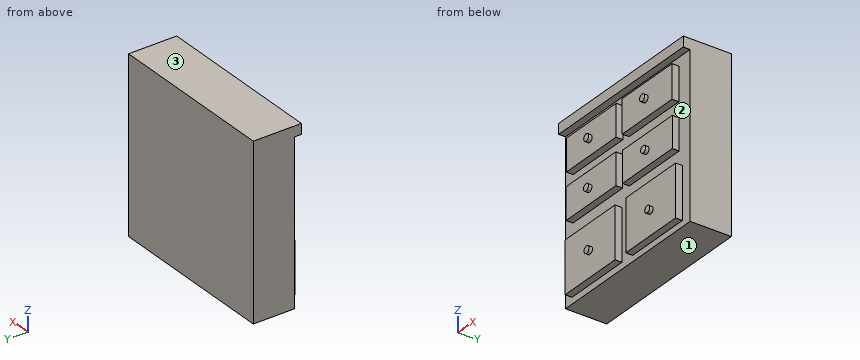
```python
from build123d import *

# Parameters (mm, degrees)
F0_W      = 50
F0_H      = 12
F1_DEPTH  = 50
F3_W      = 20
F3_H      = 9.72515
F4_DEPTH  = 2
F2_W      = 20
F2_H      = 9.250753
F5_DEPTH  = 2
F6_W      = 19.959261
F6_H      = 9.224868
F7_DEPTH  = 2
F8_W      = 20
F8_H      = 9.057143
F9_DEPTH  = 2
F10_W     = 20
F10_H     = 15
F11_DEPTH = 2
F12_W     = 20
F12_H     = 15
F13_DEPTH = 2
F14_R     = 1
F15_DEPTH = 1
F16_W     = 50
F16_H     = 3
F17_DEPTH = 2
F18_R     = 1
F19_DEPTH = 1
F20_R     = 1
F21_DEPTH = 1
F22_R     = 1
F23_DEPTH = 1
F24_R     = 1
F25_DEPTH = 1


with BuildPart() as f1:
    # F0 (on Top) → F1 (new body)
    with BuildSketch(Plane.XY):
        with Locations((25, 6)):
            Rectangle(F0_W, F0_H)
    extrude(amount=F1_DEPTH)

    # F3 (on face) → F4 (join)
    with BuildSketch(Plane.XZ):
        with Locations((35.493044, 39.7308)):
            Rectangle(F3_W, F3_H)
    extrude(amount=F4_DEPTH)

    # F2 (on face) → F5 (join)
    with BuildSketch(Plane.XZ):
        with Locations((13.077754, 39.849401)):
            Rectangle(F2_W, F2_H)
    extrude(amount=F5_DEPTH)

    # F6 (on face) → F7 (join)
    with BuildSketch(Plane.XZ):
        with Locations((12.97327, 26.628648)):
            Rectangle(F6_W, F6_H)
    extrude(amount=F7_DEPTH)

    # F8 (on face) → F9 (join)
    with BuildSketch(Plane.XZ):
        with Locations((35.595761, 25.873886)):
            Rectangle(F8_W, F8_H)
    extrude(amount=F9_DEPTH)

    # F10 (on face) → F11 (join)
    with BuildSketch(Plane.XZ):
        with Locations((12.617452, 9.389227)):
            Rectangle(F10_W, F10_H)
    extrude(amount=F11_DEPTH)

    # F12 (on face) → F13 (join)
    with BuildSketch(Plane.XZ):
        with Locations((36.937559, 9.221502)):
            Rectangle(F12_W, F12_H)
    extrude(amount=F13_DEPTH)

    # F14 (on face) → F15 (join)
    with BuildSketch(Plane.XZ.offset(2)):
        with Locations((12.452937, 39.849401)):
            Circle(F14_R)
    extrude(amount=F15_DEPTH)

    # F16 (on face) → F17 (join)
    with BuildSketch(Plane.XZ):
        with Locations((25, 48.5)):
            Rectangle(F16_W, F16_H)
    extrude(amount=F17_DEPTH)

    # F18 (on face) → F19 (join)
    with BuildSketch(Plane.XZ.offset(2)):
        with Locations((34.871425, 40.019318)):
            Circle(F18_R)
    extrude(amount=F19_DEPTH)

    # F20 (on face) → F21 (join)
    with BuildSketch(Plane.XZ.offset(2)):
        with Locations((12.349669, 26.287466)):
            Circle(F20_R)
    extrude(amount=F21_DEPTH)

    # F22 (on face) → F23 (join)
    with BuildSketch(Plane.XZ.offset(2)):
        with Locations((35.268549, 25.72331)):
            Circle(F22_R)
    extrude(amount=F23_DEPTH)

    # F24 (on face) → F25 (join)
    with BuildSketch(Plane.XZ.offset(2)):
        with Locations((12.578998, 9.153273)):
            Circle(F24_R)
        with Locations((36.913071, 8.554894)):
            Circle(F24_R)
    extrude(amount=F25_DEPTH)


solid = f1.part
```
Model file for the job. Use its own axes, mm. Face numbers are marked on the shaded views. Give positions to 0.01 mm unless a question says otherwise; leave off trailing zeros. Write each loop counter-clockwise with the first axis right and the second up, starting at its lowest first coordinate (ties: lowest second). Pieces come first, ordered by that corner, then holes. Notation, with made-up numbers: M 82,-31 L 117,-31 A27 cw 117,0 Z; hole C -36.5,46.5 d10. An arc over 180 degrees is marked long. Use a Markdown table: item, result.
1) Pull direction Z, two halves, no side cores. Call the marked faces 1, 2 and 3: +Z half, -Z half, draft (parallel to the pull), parting line (faces both ways), or undercut.
Responses:
| item | result |
|---|---|
| face 1 | -Z half |
| face 2 | undercut |
| face 3 | +Z half |
2) Cut at D-D (x = 35). List the corners of the cut face in (y, z), and give its area (3 significant figures).
Responses:
| item | result |
|---|---|
| outline | M -3,24.76 L -2,24.76 L -2,21.35 L 0,21.35 L 0,16.72 L -2,16.72 L -2,1.72 L 0,1.72 L 0,0 L 12,0 L 12,50 L -2,50 L -2,47 L 0,47 L 0,44.59 L -2,44.59 L -2,41.01 L -3,41.01 L -3,39.03 L -2,39.03 L -2,34.87 L 0,34.87 L 0,30.4 L -2,30.4 L -2,26.69 L -3,26.69 Z |
| area | 677 mm2 |
3) Cut at C-C (z = 45.5). List the corners of the cut face in (x, y).
Responses:
| item | result |
|---|---|
| outline | M 0,0 L 50,0 L 50,12 L 0,12 Z |
4) Pin check, flat tips, straight feed: pin 1 (2 mm diameter, centred on x = 15, y = -1.5, fed in from -Z); pin 2 (1 mm diameter, centred on x = 26, z = 16.5, fed in from -Y); pin 3 (1 mm diameter, centred on y = -1, z = 8.5, fed in from +X). Stop position of each tip, or through.
Responses:
| item | result |
|---|---|
| pin 1 | stops at z = 1.89 |
| pin 2 | stops at y = 0 |
| pin 3 | stops at x = 46.94 |
5) Cut at A-A (z = 37.5). List the corners of the cut face in (x, y), and give its area (3 significant figures).
Responses:
| item | result |
|---|---|
| outline | M 0,0 L 3.08,0 L 3.08,-2 L 23.08,-2 L 23.08,0 L 25.49,0 L 25.49,-2 L 45.49,-2 L 45.49,0 L 50,0 L 50,12 L 0,12 Z |
| area | 680 mm2 |
6) Cut at B-B (x = 8.5). List the corners of the cut face in (y, z).
Responses:
| item | result |
|---|---|
| outline | M -2,1.89 L 0,1.89 L 0,0 L 12,0 L 12,50 L -2,50 L -2,47 L 0,47 L 0,44.47 L -2,44.47 L -2,35.22 L 0,35.22 L 0,31.24 L -2,31.24 L -2,22.02 L 0,22.02 L 0,16.89 L -2,16.89 Z |
7) Drill centre lines: line 1 (Z direction, x = 37, y = -1); line 2 (Y direction, x = 29, z = 11); line 3 (Y direction, x = 6, z = 18). Where is each one in solid material? Low to high. Write a range as from..to.
Responses:
| item | result |
|---|---|
| line 1 | z = 1.72..16.72, 21.35..30.4, 34.87..44.59, 47..50 |
| line 2 | y = -2..12 |
| line 3 | y = 0..12 |
